For this review, take the finished solid that the model builds, in its own axes (mm). Face numbers are marked on the shaded views. A direction names the side the tool comes from. Coordinates: 2 decimals unless noted, no trailing zeros. Order: outer loops, then holes, each group sorted by start corner. A loop starts at its lowest first (then second) coordinate and runs counter-clockwise, first axis right, second up. Notation, with made-up numbers: (-13, 79) -> (21, 79) arc R19 cw to (21, 87) -> close; hole circle Ø4 at (86.5, 9.5). An arc over 180 degrees is marked (long way). Return JSON: item names as keys, results as strings. Group by question number.
Item 1: Take a section at B-B (y = 5). Write out the cut boundary in (x, z), then the cut area to 3 significant figures.
Item 2: Take a section at D-D (y = -10.5). Write out the cut boundary in (x, z), then the cut area to 3 significant figures.
Item 3: Insertion check: pin 1 (1.5 mm diameter, centred on x = -10.5, z = 13.5, fed in from -Y); pin 2 (12 mm diameter, centred on x = 8.5, z = 10.5, fed in from +Y); pin 3 (1.5 mm diameter, centred on x = 1, y = 0.5, fed in from +Z); pin 4 (1.9 mm diameter, centred on x = 0, y = -5, fed in from +Z). Each pin has a flat end and moves straight along its axis. Give the tip position at first contact, or say it passes through.
Item 4: For line 1 along X through (y, z) = (4, 23); line 2 along Y through (x, z) = (0, -1.45); line 3 along Z through (x, y) = (-11, 4.5), list the stretches that pass through material, from the lowest coordinate up.
Item 5: Machinability: for the marked faces 4 and 5, which of the approach directions +Z, -Z, +X, -X, +Y, -Y give a long, thin tool a straight path to every point of the face, cutting with its end or side? Answer none if there is none.
Item 6: Take a section at C-C (x = 4). Write out the cut boundary in (y, z), then the cut area to 3 significant figures.
Item 7: Take a section at A-A (z = 27.5). Write out the cut boundary in (x, y), then the cut area to 3 significant figures.
Item 8: Draft analysis for pull direction X (two halves, no side actions). For the marked faces 1, 2 and 3, state which applies: +X half, -X half, draft (parallel to the pull), parting line (faces both ways), or undercut.
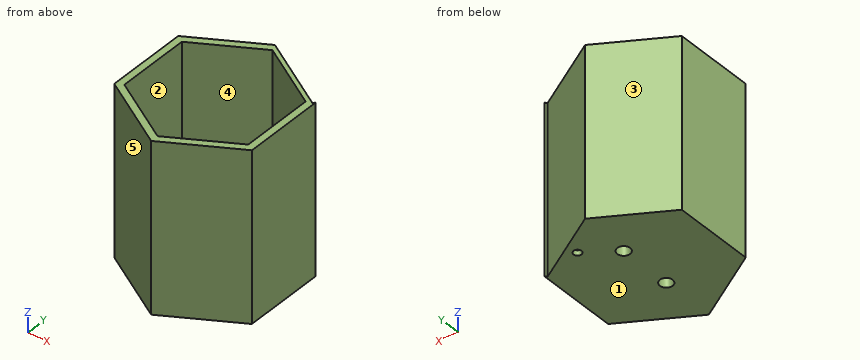
```python
from build123d import *

# Parameters (mm, degrees)
PAD_DEPTH       = 30
PAD001_DEPTH    = 2
SKETCH002_R     = 0.739951
POCKET_DEPTH    = 1
SKETCH003_R     = 1.2
POCKET001_DEPTH = 5


with BuildPart() as part:
    # Sketch → Pad (new body)
    with BuildSketch(Plane.XY):
        Polygon((-0.50397, 14.713397), (-12.984903, 7.508821), (-12.99, -7.5), (0, -14.99967), (12.99, -7.5), (12.99, 7.5), (12.74, 7.066987), align=None)
        Polygon((0, 13.49967), (-11.691057, 6.749835), (-11.691057, -6.749835), (0, -13.49967), (11.691057, -6.749835), (11.691057, 6.749835), align=None, mode=Mode.SUBTRACT)
    extrude(amount=PAD_DEPTH)

    # Sketch001 (on Face14 of Pad) → Pad001 (join)
    with BuildSketch(Plane(origin=(0, 0, 0), x_dir=(1, 0, 0), z_dir=(0, 0, -1))):
        Polygon((0, 14.99967), (12.99, 7.5), (12.99, -7.5), (12.74, -7.066987), (-0.50397, -14.713397), (-12.984903, -7.508821), (-12.99, 7.5), align=None)
    extrude(amount=PAD001_DEPTH)

    # Sketch002 (on Face10 of Pad001) → Pocket (cut)
    with BuildSketch(Plane(origin=(0, 0, -2), x_dir=(1, 0, 0), z_dir=(0, 0, -1))):
        with Locations((5.572448, -8.92072)):
            Circle(SKETCH002_R)
    extrude(amount=-POCKET_DEPTH, mode=Mode.SUBTRACT)

    # Sketch003 (on Face10 of Pocket) → Pocket001 (cut)
    with BuildSketch(Plane(origin=(0, 0, -2), x_dir=(1, 0, 0), z_dir=(0, 0, -1))):
        with Locations((0, 5)):
            Circle(SKETCH003_R)
        with Locations((0, -5)):
            Circle(SKETCH003_R)
    extrude(amount=-POCKET001_DEPTH, mode=Mode.SUBTRACT)


solid = part.part
```
Findings below:
{
 "1": {"outline": "(-12.99, -2) -> (-1.2, -2) -> (-1.2, 0) -> (-11.69, 0) -> (-11.69, 30) -> (-12.99, 30) -> close; (1.2, -2) -> (12.99, -2) -> (12.99, 30) -> (11.69, 30) -> (11.69, 0) -> (1.2, 0) -> close", "area": "125 mm2"},
 "2": {"outline": "(-7.79, -2) -> (7.79, -2) -> (7.79, 30) -> (5.2, 30) -> (5.2, 0) -> (-5.2, 0) -> (-5.2, 30) -> (-7.79, 30) -> close", "area": "187 mm2"},
 "3": {"pin 1": "stops at y = -9.37", "pin 2": "stops at y = 12.98", "pin 3": "stops at z = 0", "pin 4": "passes through"},
 "4": {"line 1": "x = -12.99 to -11.69, 11.69 to 12.99", "line 2": "y = -15 to -6.2, -3.8 to 3.8, 6.2 to 14.42", "line 3": "z = -2 to 0"},
 "5": {"face 4": "+Z", "face 5": "+Z, -Z, -X, -Y"},
 "6": {"outline": "(-12.69, -2) -> (12.11, -2) -> (12.11, 30) -> (11.19, 30) -> (11.19, 0) -> (-11.19, 0) -> (-11.19, 30) -> (-12.69, 30) -> close", "area": "122 mm2"},
 "7": {"outline": "(-12.99, -7.5) -> (0, -15) -> (12.99, -7.5) -> (12.99, 7.5) -> (12.74, 7.07) -> (-0.5, 14.71) -> (-12.98, 7.51) -> close; hole (-11.69, -6.75) -> (0, -13.5) -> (11.69, -6.75) -> (11.69, 6.75) -> (0, 13.5) -> (-11.69, 6.75) -> close", "area": "104 mm2"},
 "8": {"face 1": "draft", "face 2": "undercut", "face 3": "-X half"}
}
